Here's the drawing with two shaded views (mm, measured from the low corner). I have some questions. A direction names the side the tool comes from. Give positions to 0.01 mm unless a question says otherwise; leave off trailing zeros. Order: outer loops, then holes, each group sorted by start corner. A loop starts at its lowest first (then second) coordinate and runs counter-clockwise, first axis right, second up. Notation, with made-up numbers: M 27.25,-17.5 L 69.25,-17.5 A17 cw 69.25,-1.5 Z; hole C -13.75,-37.5 d5. An arc over 180 degrees is marked long. One line per question, with ' | ' between items. Start each with the question number.
1) If we section it at D-D, the plane x = 75: Please give me the cut outline in (y, z).
2) If we section it at B-B, the plane x = 120: Please give me the cut outline in (y, z), plus the area to 3 significant figures.
3) Thinking about a two-plate mould opening in X: for the marked faces 1 and 2, which applies, +X half, -X half, draft (parallel to the pull), parting line (faces both ways), or undercut?
4) If we section it at C-C, the plane z = 75: Please give me the cut outline in (x, y), plus the area to 3 significant figures.
5) I'm going to push flat-ended pins straight in: pin 1 Ø1.2 at (y, z) = (15.5, 90.5) entering from -X; pin 2 Ø4.5 at (x, z) = (30, 40) entering from +Y; pin 3 Ø6 at (y, z) = (6, 31.5) entering from +X. Where does each tip first touch, or does it pass through?
6) If we section it at A-A, the plane y = 10.5: Please give me the cut outline in (x, z), plus the area to 3 significant figures.
7) For the marked faces 3 and 4, which set-ups out of +Z, -Z, +X, -X, +Y, -Y let a thin tool reach every point of the face, with its end or its side?
8) Please list where these lines run through material, in increasing order: line 1 along X through (y, z) = (2.8, 75); line 2 along X through (y, z) = (15.25, 120); line 3 along X through (y, z) = (2.65, 40). Write a range as [from, to].
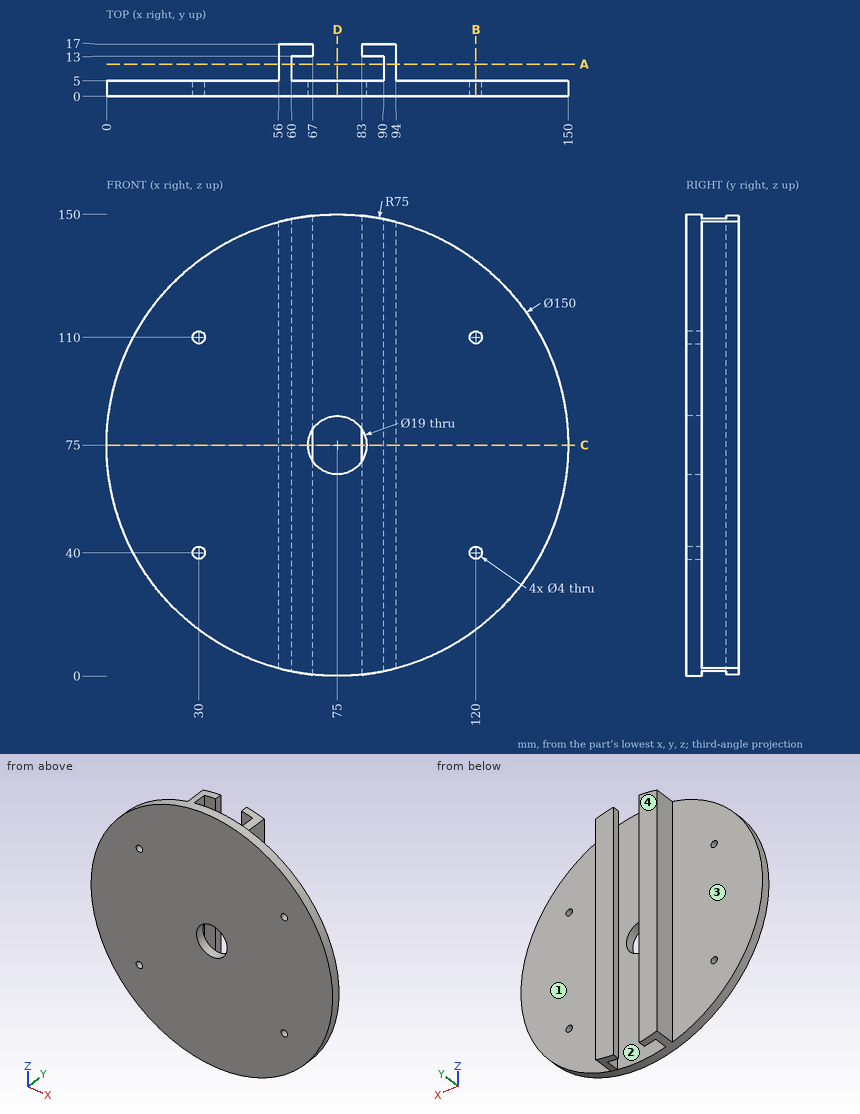
Results found:
1) outline: M 0,0 L 5,0 L 5,65.5 L 0,65.5 Z; M 0,84.5 L 5,84.5 L 5,150 L 0,150 Z
2) outline: M 0,15 L 5,15 L 5,38 L 0,38 Z; M 0,42 L 5,42 L 5,108 L 0,108 Z; M 0,112 L 5,112 L 5,135 L 0,135 Z | area: 560 mm²
3) face 1: draft | face 2: undercut
4) outline: M 0,0 L 65.5,0 L 65.5,5 L 60,5 L 60,13 L 67,13 L 67,17 L 56,17 L 56,5 L 0,5 Z; M 83,13 L 90,13 L 90,5 L 84.5,5 L 84.5,0 L 150,0 L 150,5 L 94,5 L 94,17 L 83,17 Z | area: 807 mm²
5) pin 1: stops at x = 56 | pin 2: stops at y = 5 | pin 3: stops at x = 138.01
6) outline: M 56,2.45 A75 ccw 60,1.52 L 60,148.48 A75 ccw 56,147.55 Z; M 90,1.52 A75 ccw 94,2.45 L 94,147.55 A75 ccw 90,148.48 Z | area: 1,170 mm²
7) face 3: +Z, -Z, -X, +Y | face 4: +Z, -Z, +X, -X, +Y
8) line 1: x = [0, 65.5], [84.5, 150] | line 2: x = [56, 67], [83, 94] | line 3: x = [8.67, 28], [32, 118], [122, 141.33]
